```python
from build123d import *

# Parameters (mm, degrees)
BOX001_W          = 20
BOX001_H          = 2
BOX001_DEPTH      = 10
BOX_W             = 2
BOX_H             = 20
BOX_DEPTH         = 10
CYLINDER002_R     = 4
CYLINDER002_DEPTH = 10
TORUS_R           = 1
CYLINDER001_R     = 6.5
CYLINDER001_DEPTH = 10
CYLINDER_R        = 7.7
CYLINDER_DEPTH    = 4
CHAMFER_SIZE      = 1


with BuildPart() as cube001:
    # Box001 → Box001 (new body)
    with BuildSketch(Plane(origin=(-10, -1, 4), x_dir=(1, 0, 0), z_dir=(0, 0, 1))):
        with Locations((10, 1)):
            Rectangle(BOX001_W, BOX001_H)
    extrude(amount=BOX001_DEPTH)


with BuildPart() as cube:
    # Box → Box (new body)
    with BuildSketch(Plane(origin=(-1, -10, 4), x_dir=(1, 0, 0), z_dir=(0, 0, 1))):
        with Locations((1, 10)):
            Rectangle(BOX_W, BOX_H)
    extrude(amount=BOX_DEPTH)


with BuildPart() as fusion002:
    # Cylinder002 → Cylinder002 (new body)
    with BuildSketch(Plane.XY.offset(4)):
        Circle(CYLINDER002_R)
    extrude(amount=CYLINDER002_DEPTH)

    # Fusion002: union Cube001, Cube
    add(cube001.part)
    add(cube.part)


with BuildPart() as torus:
    # Torus → Torus (revolve)
    with BuildSketch(Plane(origin=(0, 0, 11), x_dir=(1, 0, 0), z_dir=(0, -1, 0))):
        with Locations((6, 0)):
            Circle(TORUS_R)
    revolve(axis=Axis((0, 0, 11), (0, 0, 1)))


with BuildPart() as cylinder001:
    # Cylinder001 → Cylinder001 (new body)
    with BuildSketch(Plane.XY.offset(2)):
        Circle(CYLINDER001_R)
    extrude(amount=CYLINDER001_DEPTH)


with BuildPart() as cylinder:
    # Cylinder → Cylinder (new body)
    with BuildSketch(Plane.XY):
        Circle(CYLINDER_R)
    extrude(amount=CYLINDER_DEPTH)


with BuildPart() as obj1:
    # Sphere → Sphere (revolve)
    with BuildSketch(Plane(origin=(0, 0, 20), x_dir=(1, 0, 0), z_dir=(0, -1, 0))):
        with BuildLine():
            ThreePointArc((0, -20), (20, 0), (0, 20))
            Line((0, 20), (0, -20))
        make_face()
    revolve(axis=Axis((0, 0, 20), (0, 0, 1)))

    # Common: intersect Cylinder
    add(cylinder.part, mode=Mode.INTERSECT)

    # Fusion: union Cylinder001
    add(cylinder001.part)

    # Chamfer
    chamfer_edges = [obj1.edges().sort_by_distance(p)[0] for p in [
        (-6.5, 0, 12),
    ]]
    chamfer(chamfer_edges, length=CHAMFER_SIZE)

    # Fusion001: union Torus
    add(torus.part)

    # Cut: cut Fusion002
    add(fusion002.part, mode=Mode.SUBTRACT)


solid = obj1.part
```
CAD build for the part. Positions are in the model's coordinates, mm. A direction names the side the tool comes from. Give positions to 0.01 mm unless a question says otherwise; leave off trailing zeros. Order: outer loops, then holes, each group sorted by start corner. A loop starts at its lowest first (then second) coordinate and runs counter-clockwise, first axis right, second up.
(1) Tool access for faces 1 (the cylindrical face through (4.637, 4.555, 7.024)), 2 (the flat face through (-5, -1, 8)), 3 (the cylindrical face through (-2.849, -2.807, 7.944)), 4 (the flat face through (-1, -5, 8)): list every direction of +Z, -Z, +X, -X, +Y, -Y with a clear straight run to the whole face (end or side of a thin tool).
(2) Flat gauge pins, fed straight in: pin 1 (2.5 mm diameter, centred on x = 5.5, z = 6, fed in from -Y); pin 2 (3 mm diameter, centred on x = 0.5, y = -1.5, fed in from +Z); pin 3 (4 mm diameter, centred on y = 1, z = 10.5, fed in from -X); pin 4 (5 mm diameter, centred on x = 1, y = 1.5, fed in from +Z). Where does each tip first touch, or does it go through?
(3) Saw through at D-D, the plane z = 11.25. Give the cut face in (x, y).
(4) Mould opens along X. For faces 5 (the cylindrical face through (2.849, 2.807, 7.944)), 6 (the cylindrical face through (-4.637, -4.555, 7.024)), 7 (the flat face through (5, -1, 8)), 8 (the cylindrical face through (2.807, -2.849, 7.944)) say: released by +X, released by -X, zero draft, split by the parting line, or undercut.
(5) Saw through at B-B, the plane x = 0. Give the cut face in (y, z), then the cut area to 3 significant figures.
(6) Drill centre lines: L1, parallel to Y at x = -6, z = 6.75; L2, parallel to X at y = -3, z = 6.75; L3, parallel to Y at x = 2, z = 9.25. Where is each one in solid material? Low to high.
(7) Saw through at A-A, the plane z = 7.5. Give the cut face in (x, y).
Results found:
1. face 1: +X, +Y
1. face 2: +Z, +X, -X
1. face 3: +Z
1. face 4: +Z, +Y, -Y
2. pin 1: stops at y = -4.92
2. pin 2: stops at z = 4
2. pin 3: stops at x = -6.93
2. pin 4: stops at z = 12
3. outline: (-6.9, -1) arc R6.97 ccw to (-1, -6.9) - (-1, -3.87) arc R4 cw to (-3.87, -1) - close; (-6.9, 1) - (-3.87, 1) arc R4 cw to (-1, 3.87) - (-1, 6.9) arc R6.97 ccw to start; (1, -6.9) arc R6.97 ccw to (6.9, -1) - (3.87, -1) arc R4 cw to (1, -3.87) - close; (1, 3.87) arc R4 cw to (3.87, 1) - (6.9, 1) arc R6.97 ccw to (1, 6.9) - close
4. face 5: undercut
4. face 6: released by -X
4. face 7: zero draft
4. face 8: undercut
5. outline: (-7.7, 1.54) arc R20 ccw to (7.7, 1.54) - (7.7, 4) - (-7.7, 4) - close
5. area: 53.8 mm2
6. L1: y = -2.5 to -1, 1 to 2.5
6. L2: x = -5.77 to -2.65, 2.65 to 5.77
6. L3: y = -6.18 to -3.46, 3.46 to 6.18
7. outline: (-6.42, -1) arc R6.5 ccw to (-1, -6.42) - (-1, -3.87) arc R4 cw to (-3.87, -1) - close; (-6.42, 1) - (-3.87, 1) arc R4 cw to (-1, 3.87) - (-1, 6.42) arc R6.5 ccw to start; (1, -6.42) arc R6.5 ccw to (6.42, -1) - (3.87, -1) arc R4 cw to (1, -3.87) - close; (1, 3.87) arc R4 cw to (3.87, 1) - (6.42, 1) arc R6.5 ccw to (1, 6.42) - close
